from build123d import *

# Parameters (mm, degrees)
F1_DEPTH = 25.4
F2_R     = 3.96875
F3_DEPTH = 63.501
F4_R     = 6.35
F5_DEPTH = 50.801
F6_SIZE  = 1.016


with BuildPart() as f1:
    # F0 (on Top) → F1 (new body)
    with BuildSketch(Plane.XY):
        Polygon((-44.45, 0), (0, 0), (0, -31.75), (19.05, -31.75), (19.05, 19.05), (-44.45, 19.05), align=None)
    extrude(amount=F1_DEPTH)

    # F2 (on face) → F3 (cut, through all)
    with BuildSketch(Plane.YZ.offset(19.05)):
        with BuildLine():
            ThreePointArc((-28.575, 7.200738686), (-31.75, 12.7), (-28.575, 18.199261314))
            Line((-28.575, 18.199261314), (-16.1029547439, 25.4))
            Line((-16.1029547439, 25.4), (-16.1029547439, 30.48))
            Line((-16.1029547439, 30.48), (-41.5029547439, 30.48))
            Line((-41.5029547439, 30.48), (-41.5029547439, -5.08))
            Line((-41.5029547439, -5.08), (-16.1029547439, -5.08))
            Line((-16.1029547439, -5.08), (-16.1029547439, 0))
            Line((-16.1029547439, 0), (-28.575, 7.200738686))
        make_face()
        with Locations((-25.4, 12.7)):
            Circle(F2_R)
    extrude(amount=-F3_DEPTH, mode=Mode.SUBTRACT)

    # F4 (on face) → F5 (cut, through all)
    with BuildSketch(Plane(origin=(0, 19.05, 0), x_dir=(-1, 0, 0), z_dir=(0, 1, 0))):
        with Locations((25.4, 12.7)):
            Circle(F4_R)
    extrude(amount=-F5_DEPTH, mode=Mode.SUBTRACT)

    # F6
    f6_edges = [f1.edges().sort_by_distance(p)[0] for p in [
        (19.05, -29.36875, 12.7),
        (9.525, -21.43125, 12.7),
        (0, -29.36875, 12.7),
    ]]
    chamfer(f6_edges, length=F6_SIZE)


solid = f1.part
Can you work these out from the model? Positions are in its coordinate system, mm. A direction names the side the tool comes from. Give positions to 0.01 mm unless a question says otherwise; leave off trailing zeros. Loops run counter-clockwise (first coordinate to the right, second up) from the corner with the lowest first, then second, coordinate; pieces in that order, holes last. Notation, with made-up numbers: M 39,-6.75 L 96,-6.75 A14 cw 96,-2.75 Z; hole C 36.25,-17.5 d8. An arc over 180 degrees is marked long. One line per item, written item: value. Start each with the question number.
1) If we section it at A-A, the plane x = -25.4: Write out the boundary of the cut face in (y, z).
2) I'm going to push flat-ended pins straight in: pin 1 (12 mm diameter, centred on x = -28.5, y = 6, fed in from -Z); pin 2 (7.5 mm diameter, centred on x = -25.4, z = 12.7, fed in from -Y); pin 3 (4 mm diameter, centred on y = -20.5, z = 6, fed in from -X). Where does each tip first touch, or does it pass through?
3) Thinking about a two-plate mould opening in Y: for faces 3 (the face through (9.644, -28.549, 10.285)), 4 (the face through (-6, 6, 0)), 5 (the face through (9.66, -22.25, 3.55)), which applies, +Y half, -Y half, draft (parallel to the pull), parting line (faces both ways), or undercut?
4) If we section it at C-C, the plane y = -25.4: Write out the boundary of the cut face in (x, z), and give its area (3 significant figures).
5) If we section it at B-B, the plane z = 12.7: Write out the boundary of the cut face in (x, y).
6) On a 3-axis mill with a long thin cutter (end or side, diameter ignored), from which of +Z, -Z, +X, -X, +Y, -Y can I reach the whole of each face in a straight line? I mean faces 1 (the face through (-18, 0, 13)), 2 (the face through (19.05, -1, 13)). Say none if no direction works.
7) If I drill on line 1 (Z direction, x = -25.4, y = 13.75); line 2 (Y direction, x = -23, z = 24); line 3 (Y direction, x = 4, z = 2.5), over which ranges is the centre line in solid material (lowest first)? Write a range as [from, to].
Completed:
1. outline: M 0,0 L 19.05,0 L 19.05,6.35 L 0,6.35 Z; M 0,19.05 L 19.05,19.05 L 19.05,25.4 L 0,25.4 Z
2. pin 1: stops at z = 0
2. pin 2: passes through
2. pin 3: stops at x = 0
3. face 3: undercut
3. face 4: draft
3. face 5: -Y half
4. outline: M 0,5.37 L 19.05,5.37 L 19.05,7.72 L 18.03,8.73 L 1.02,8.73 L 0,7.72 Z; M 0,17.68 L 1.02,16.67 L 18.03,16.67 L 19.05,17.68 L 19.05,20.03 L 0,20.03 Z
4. area: 126 mm^2
5. outline: M -44.45,0 L -31.75,0 L -31.75,19.05 L -44.45,19.05 Z; M -19.05,0 L 0,0 L 0,-20.42 L 1.02,-21.43 L 18.03,-21.43 L 19.05,-20.42 L 19.05,19.05 L -19.05,19.05 Z; M 0,-31.75 L 19.05,-31.75 L 19.05,-30.38 L 18.03,-29.37 L 1.02,-29.37 L 0,-30.38 Z
6. face 1: +Z, -Z, -X, -Y
6. face 2: +Z, -Z, +X, +Y, -Y
7. line 1: z = [0, 6.35], [19.05, 25.4]
7. line 2: y = [0, 19.05]
7. line 3: y = [-20.43, 19.05]
